Source: CAD feature listing. Evaluate the final solid. Frame: model axes, mm. A direction names the side the tool comes from. Coordinates: 2 decimals unless noted, no trailing zeros. Order: outer loops, then holes, each group sorted by start corner. A loop starts at its lowest first (then second) coordinate and runs counter-clockwise, first axis right, second up.
Item 1: Section D-D on z = 4.4. Return the cut outline in (x, y).
Item 2: Ray query, line 1 (Z direction, x = 2.35, y = 0.6); line 2 (Y direction, x = 1.2, z = 2.65). Return the intervals inside material, ascending.
Item 3: Reachability of faces 1 (the flat face through (-1.5, 0, 1)), 2 (the flat face through (0, 1.5, 1)), 3 (the flat face through (1.5, 0, 1)), 4 (the flat face through (0, -1.5, 1)) from +Z, -Z, +X, -X, +Y, -Y: full face, straight path, thin tool, end or side. Return the list, or none.
Item 4: Contact query for flat-ended pins moving along their axis: P1, Ø1, axis at x = 0.5, z = 4, coming from the -Y side; P2, Ø0.9, axis at y = 0, z = 1, coming from the +X side; P3, Ø1.5, axis at x = 0.5, z = 2, coming from the -Y side. Output: stop coordinate, or through.
Item 5: Section A-A on y = 0. Return the cut outline in (x, z).
Item 6: Section C-C on z = 1.2. Return the cut outline in (x, y), then the cut area to 3 significant figures.
from build123d import *

# Parameters (mm, degrees)
BOSS_EXTRUDE1_DEPTH = 3
SKETCH2_R           = 2.5
BOSS_EXTRUDE2_DEPTH = 3


with BuildPart() as part:
    # Sketch1 → Boss-Extrude1 (new body)
    with BuildSketch(Plane.XY):
        Polygon((-1.5, 0), (-1.5, 1.5), (1.5, 1.5), (1.5, -1.5), (-1.5, -1.5), align=None)
    extrude(amount=BOSS_EXTRUDE1_DEPTH)

    # Sketch2 → Boss-Extrude2 (add)
    with BuildSketch(Plane.XY.offset(3)):
        Circle(SKETCH2_R)
    extrude(amount=BOSS_EXTRUDE2_DEPTH)


solid = part.part
Answer list:
1. outline: circle Ø5 at (0, 0)
2. line 1: z = 3 to 6
2. line 2: y = -1.5 to 1.5
3. face 1: -Z, -X, +Y, -Y
3. face 2: -Z, +X, -X, +Y
3. face 3: -Z, +X, +Y, -Y
3. face 4: -Z, +X, -X, -Y
4. P1: stops at y = -2.5
4. P2: stops at x = 1.5
4. P3: stops at y = -1.5
5. outline: (-2.5, 3) - (-1.5, 3) - (-1.5, 0) - (1.5, 0) - (1.5, 3) - (2.5, 3) - (2.5, 6) - (-2.5, 6) - close
6. outline: (-1.5, -1.5) - (1.5, -1.5) - (1.5, 1.5) - (-1.5, 1.5) - close
6. area: 9.00 mm2
